Geometry: final body of the model. Coordinates: model frame, mm. A direction names the side the tool comes from. Coordinates: 2 decimals unless noted, no trailing zeros. Loops run counter-clockwise (first coordinate to the right, second up) from the corner with the lowest first, then second, coordinate; pieces in that order, holes last. Notation, with made-up numbers: M 86,-38.5 L 111,-38.5 A13 cw 111,-32.5 Z; hole C -12,70 d3. An arc over 180 degrees is marked long. Write item = value, one per line. Start each with the question number.
```python
from build123d import *

# Parameters (mm, degrees)
SKETCH1_R           = 15.5
SKETCH1_R_2         = 1
SKETCH1_W           = 8
SKETCH1_H           = 6
BOSS_EXTRUDE1_DEPTH = 2


with BuildPart() as part:
    # Sketch1 → Boss-Extrude1 (new body)
    with BuildSketch(Plane(origin=(0, 0, 0), x_dir=(0, -1, 0), z_dir=(0, 0, 1))):
        Circle(SKETCH1_R)
        with Locations((6.97426488, 10.435972737)):
            Circle(SKETCH1_R_2, mode=Mode.SUBTRACT)
        with Locations((-8.02573512, -8.580948715)):
            Circle(SKETCH1_R_2, mode=Mode.SUBTRACT)
        with Locations((-0.025715642, 10.93618237)):
            Rectangle(SKETCH1_W, SKETCH1_H, mode=Mode.SUBTRACT)
    extrude(amount=BOSS_EXTRUDE1_DEPTH)


solid = part.part
```
Item 1: First-contact query: pin 1 (1.8 mm diameter, centred on x = 10.44, y = -6.97, fed in from -Z). Flat tip, straight axial feed; report the tip coordinate or a pass-through.
Item 2: Section query A-A (y = 0). Return the cut outline in (x, z), plus the area to 3 significant figures.
Item 3: Line query: line 1 (Y direction, x = 10, z = 0.75); line 2 (Y direction, x = 13, z = 1.5); line 3 (X direction, y = -7, z = 0.1). Output: solid intervals per line, ascending. Write a range as from..to.
Item 4: Pull-direction query (X, two-part tool) for faces 3 (the flat face through (0, 0, 2)), 4 (the cylindrical face through (11.28, -7.51, 0.99)), 5 (the cylindrical face through (15.368, 2.018, 0.986)); classes: released by +X, released by -X, zero draft, split by the parting line, or undercut.
Item 5: Reachability of faces 1 (the flat face through (0, 0, 0)), 2 (the flat face through (7.936, 0, 1)) from +Z, -Z, +X, -X, +Y, -Y: full face, straight path, thin tool, end or side. Return the list, or none.
Item 6: Section query D-D (y = -7). Return the cut outline in (x, z).
Item 7: Section query B-B (z = 1.5). Return the cut outline in (x, y), plus the area to 3 significant figures.
Item 8: Section query C-C (x = -7). Return the cut outline in (y, z).
Verdict:
q1.pin_1 = through
q2.outline = M -15.5,0 L 7.94,0 L 7.94,2 L -15.5,2 Z; M 13.94,0 L 15.5,0 L 15.5,2 L 13.94,2 Z
q2.area = 50.0 mm2
q3.line_1 = -11.84..-7.87, -6.07..-3.97, 4.03..11.84
q3.line_2 = -8.44..-3.97, 4.03..8.44
q3.line_3 = -13.83..9.44, 11.44..13.83
q4.face_3 = zero draft
q4.face_4 = undercut
q4.face_5 = split by the parting line
q5.face_1 = -Z, +X, -X, +Y, -Y
q5.face_2 = +Z, -Z
q6.outline = M -13.83,0 L 9.44,0 L 9.44,2 L -13.83,2 Z; M 11.44,0 L 13.83,0 L 13.83,2 L 11.44,2 Z
q7.outline = C 0,0 d31; hole C -8.58,8.03 d2; hole M 7.94,-3.97 L 13.94,-3.97 L 13.94,4.03 L 7.94,4.03 Z; hole C 10.44,-6.97 d2
q7.area = 700 mm2
q8.outline = M -13.83,0 L 13.83,0 L 13.83,2 L -13.83,2 Z
